Verification items for the finished model (mm, model axes). A direction names the side the tool comes from. Coordinates: 2 decimals unless noted, no trailing zeros. Order: outer loops, then holes, each group sorted by start corner. A loop starts at its lowest first (then second) coordinate and runs counter-clockwise, first axis right, second up.
Q1. Depth check by flat-ended pin: P1, Ø1, axis at x = 1.5, y = -9.5, coming from the +Z side; P2, Ø6, axis at x = -9, z = 11, coming from the -Y side. Enter the tip coordinate at first touch or a pass-through.
Q2. Thickness scan on line 1 (Z direction, x = 3.5, y = -5.25); line 2 (Y direction, x = -21.5, z = 19); line 3 (X direction, y = -7.25, z = 10.5). Record the ranges inside material, lowest first.
Q3. Cross-section at D-D, the plane y = -3.5. Record the boundary of the cut face in (x, z), and give its area (3 significant figures).
Q4. Cross-section at A-A, the plane x = -25.5. Record the boundary of the cut face in (y, z), and give its area (3 significant figures).
Q5. Cross-section at B-B, the plane y = -7.75. Record the boundary of the cut face in (x, z), and give its area (3 significant figures).
Q6. Set-up check for faces 1 (the flat face through (-5, -7, 33.513)), 2 (the cylindrical face through (-4.743, -1.449, 1.528)): record each of +Z, -Z, +X, -X, +Y, -Y from which the full face is reachable in a straight line by a thin tool's end or side.
Q7. Draft check along X on faces 3 (the flat face through (-28.693, -7, 18)), 4 (the cylindrical face through (-29.784, -1.528, 18.279)), 5 (the cylindrical face through (-5.47, -9.11, 35.39)). Enter one of: pulls with the +X half, pulls with the -X half, needs draft (parallel to the pull), parting line crosses it, or undercut.
Q8. Cross-section at C-C, the plane z = 13. Record the boundary of the cut face in (x, y), and give its area (3 significant figures).
from build123d import *

# Parameters (mm, degrees)
F0_W        = 52.2474944592
F0_H        = 36.0527001321
F1_DEPTH    = 11.684
F2_T        = -2.54
F3_T1_DEPTH = 61.4527001321
F3_T3_DEPTH = 77.6474944592
F4_R        = 5.08


# Not quite as in the source:
# - a fillet or chamfer that OpenCascade refuses, or shapes differently, is made with other operations: its cross-section is extruded or revolved along the edge and cut away or added


with BuildPart() as f1:
    # F0 (on Front) → F1 (new body)
    with BuildSketch(Plane.XZ):
        with Locations((-5.1090717316, 18.0263500661)):
            Rectangle(F0_W, F0_H)
    extrude(amount=F1_DEPTH)

    # F2
    f2_openings = [f1.faces().sort_by_distance(p)[0] for p in [
        (-5.109072, -11.684, 18.02635),
    ]]
    offset(amount=F2_T, openings=f2_openings)

    # F3: fillet of radius 5.08 on 4 edges, made by hand

    # F3_s2 → F3_t1 (cut)
    with BuildSketch(Plane.XY.offset(-12.7)):
        with BuildLine():
            ThreePointArc((21.014675498, -6.604), (19.5267779464, -10.1961024484), (15.934675498, -11.684))
            Line((15.934675498, -11.684), (21.014675498, -11.684))
            Line((21.014675498, -11.684), (21.014675498, -6.604))
        make_face()
        with BuildLine():
            ThreePointArc((-31.2328189611, -6.604), (-29.7449214096, -10.1961024484), (-26.1528189611, -11.684))
            Line((-26.1528189611, -11.684), (-31.2328189611, -11.684))
            Line((-31.2328189611, -11.684), (-31.2328189611, -6.604))
        make_face()
    extrude(amount=F3_T1_DEPTH, mode=Mode.SUBTRACT)

    # F3_s4 → F3_t3 (cut)
    with BuildSketch(Plane.YZ.offset(-43.9328189611)):
        with BuildLine():
            ThreePointArc((-6.604, 36.0527001321), (-10.1961024484, 34.5648025806), (-11.684, 30.9727001321))
            Line((-11.684, 30.9727001321), (-11.684, 36.0527001321))
            Line((-11.684, 36.0527001321), (-6.604, 36.0527001321))
        make_face()
        with BuildLine():
            ThreePointArc((-6.604, 0), (-10.1961024484, 1.4878975516), (-11.684, 5.08))
            Line((-11.684, 5.08), (-11.684, 0))
            Line((-11.684, 0), (-6.604, 0))
        make_face()
    extrude(amount=F3_T3_DEPTH, mode=Mode.SUBTRACT)

    # F4
    f4_edges = [f1.edges().sort_by_distance(p)[0] for p in [
        (-5.109072, 0, 0),
        (-31.232819, 0, 18.02635),
        (-5.109072, 0, 36.0527),
        (21.014675, 0, 18.02635),
    ]]
    fillet(f4_edges, radius=F4_R)


solid = f1.part
Check values:
1. P1: stops at z = 35.45
1. P2: stops at y = -2.54
2. line 1: z = 0 to 2.54, 33.51 to 36.05
2. line 2: y = -2.54 to 0
2. line 3: x = -31.19 to -28.69, 18.47 to 20.97
3. outline: (-30.98, 0.25) - (20.76, 0.25) - (20.76, 35.8) - (-30.98, 35.8) - close; hole (-28.69, 2.54) - (18.47, 2.54) - (18.47, 33.51) - (-28.69, 33.51) - close
3. area: 379 mm2
4. outline: (-11, 2.54) arc R5.08 ccw to (-6.6, 0) - (-5.08, 0) arc R5.08 ccw to (0, 5.08) - (0, 30.97) arc R5.08 ccw to (-5.08, 36.05) - (-6.6, 36.05) arc R5.08 ccw to (-11, 33.51) - (-2.54, 33.51) - (-2.54, 2.54) - close
4. area: 117 mm2
5. outline: (-31.1, 0.13) - (20.88, 0.13) - (20.88, 35.92) - (-31.1, 35.92) - close; hole (-28.69, 2.54) - (18.47, 2.54) - (18.47, 33.51) - (-28.69, 33.51) - close
5. area: 400 mm2
6. face 1: -Y
6. face 2: -Z, +X, -X, +Y
7. face 3: undercut
7. face 4: pulls with the -X half
7. face 5: needs draft
8. outline: (-31.23, -6.6) arc R5.08 ccw to (-28.69, -11) - (-28.69, -2.54) - (18.47, -2.54) - (18.47, -11) arc R5.08 ccw to (21.01, -6.6) - (21.01, -5.08) arc R5.08 ccw to (15.93, 0) - (-26.15, 0) arc R5.08 ccw to (-31.23, -5.08) - close
8. area: 158 mm2
